The model under review builds one solid part; all positions refer to its coordinate system, in mm. Face numbers are marked on the shaded views. Coordinates: 2 decimals unless noted, no trailing zeros. Loops run counter-clockwise (first coordinate to the right, second up) from the corner with the lowest first, then second, coordinate; pieces in that order, holes last. Notation, with made-up numbers: (76.5, 54) - (91.5, 54) arc R19 cw to (91.5, 78) - close; hole circle Ø6 at (77.25, -13). An arc over 180 degrees is marked (long way). Use a Markdown table: item, result. Add a question column.
1) To check wall thickness, follow L1, parallel to Y at x = -21.25, z = -14.8; L2, parallel to Y at x = -264.45, z = -14.8; L3, parallel to X at y = 181.5, z = -10. State the ranges of each line that lie inside material, in increasing order. Write a range as [from, to].
2) Clearance check with flat-ended pins moving along their axes: pin 1 (2 mm diameter, centred on y = 182, z = -22.8, fed in from +X); pin 2 (1.1 mm diameter, centred on x = -21.5, y = 177, fed in from -Z); pin 3 (6 mm diameter, centred on x = -83.5, z = -5.5, fed in from +Y); pin 4 (12 mm diameter, centred on x = -177, y = 99.5, fed in from +Z). State where each tip first meets the part, or that it passes through.
3) Add section B-B, the plane y = 73. Give the boundary of the cut face in (x, z).
4) Add section A-A, the plane z = -35. Give the boundary of the cut face in (x, y), and give its area (3 significant figures).
5) The part is to be moulded in two halves that separate along X. For the marked faces 1, 2, 3 and 4, say which applies: pulls with the +X half, pulls with the -X half, needs draft (parallel to the pull), parting line crosses it, or undercut.
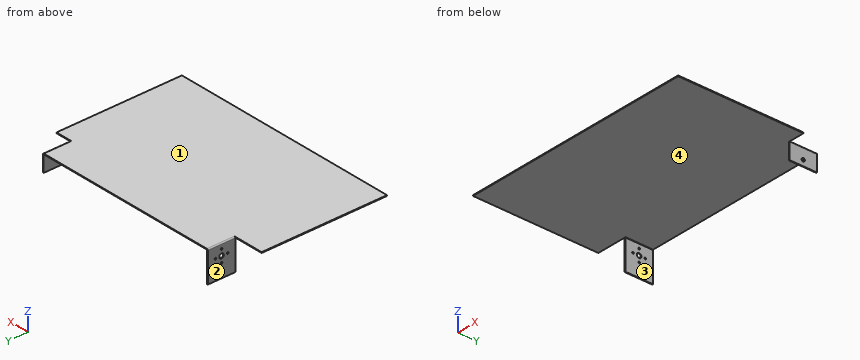
```python
from build123d import *

# Parameters (mm, degrees)
SKETCH1_W                    = 304
SKETCH1_H                    = 200
BASE_FLANGE1_DEPTH           = 1
SKETCH2_W                    = 39
SKETCH2_H                    = 36
CUT_EXTRUDE1_DEPTH           = 10
EDGE_FLANGE1_STRIP_W         = 5
EDGE_FLANGE1_STRIP_H         = 1
EDGE_FLANGE1_STRIP_CUT_DEPTH = 36
EDGE_FLANGE1_DEPTH           = 36
SKETCH9_R                    = 1.1
SKETCH9_R_2                  = 3
CUT_EXTRUDE2_DEPTH           = 10
CUT_EXTRUDE4_REACH           = 368.129
SKETCH18_W                   = 20.8
SKETCH18_H                   = 36
EDGE_FLANGE2_STRIP_W         = 5
EDGE_FLANGE2_STRIP_H         = 1
EDGE_FLANGE2_STRIP_CUT_DEPTH = 36
EDGE_FLANGE2_DEPTH           = 36
M4_CLEARANCE_HOLE2_D         = 4.3


# Sheet-metal steps are written as plain solids
with BuildPart() as part:
    # Sketch1 → Base-Flange1 (new body)
    with BuildSketch(Plane.XY):
        with Locations((-152, 100)):
            Rectangle(SKETCH1_W, SKETCH1_H)
    extrude(amount=-BASE_FLANGE1_DEPTH)

    # Sketch2 → Cut-Extrude1 (cut)
    with BuildSketch(Plane.XY):
        with Locations((-284.5, 182)):
            Rectangle(SKETCH2_W, SKETCH2_H)
    extrude(amount=-CUT_EXTRUDE1_DEPTH, mode=Mode.SUBTRACT)

    # Edge-Flange1 strip (across the edge) → Edge-Flange1 strip cut (cut)
    with BuildSketch(Plane(origin=(-265, 164, -1), x_dir=(1, 0, 0), z_dir=(0, 1, 0))):
        with Locations((-1, -0.5)):
            Rectangle(EDGE_FLANGE1_STRIP_W, EDGE_FLANGE1_STRIP_H)
    extrude(amount=EDGE_FLANGE1_STRIP_CUT_DEPTH, mode=Mode.SUBTRACT)

    # Edge-Flange1 section (across the edge) → Edge-Flange1 (add)
    with BuildSketch(Plane(origin=(-265, 164, -1), x_dir=(1, 0, 0), z_dir=(0, 1, 0))):
        with BuildLine():
            Line((0, 0.5), (0, 39.429))
            Line((0, 39.429), (1, 39.429))
            Line((1, 39.429), (1, 0.5))
            ThreePointArc((1, 0.5), (1.146446609, 0.146446609), (1.5, 0))
            Line((1.5, 0), (1.5, -1))
            ThreePointArc((1.5, -1), (0.439339828, -0.560660172), (0, 0.5))
        make_face()
    extrude(amount=EDGE_FLANGE1_DEPTH)

    # Sketch9 → Cut-Extrude2 (cut)
    with BuildSketch(Plane(origin=(-264, 0, 0), x_dir=(0, 0, -1), z_dir=(1, 0, 0))):
        with Locations((22.8, 182)):
            Circle(SKETCH9_R)
        with Locations((14.8, 190)):
            Circle(SKETCH9_R)
        with Locations((14.8, 174)):
            Circle(SKETCH9_R)
        with Locations((6.8, 182)):
            Circle(SKETCH9_R)
        with Locations((14.8, 182)):
            Circle(SKETCH9_R_2)
    extrude(amount=-CUT_EXTRUDE2_DEPTH, mode=Mode.SUBTRACT)

    # Sketch18 → Cut-Extrude4 (cut, up to next)
    with BuildSketch(Plane.XY, mode=Mode.PRIVATE) as cut_extrude4_sk1:
        with Locations((-10.4, 182)):
            Rectangle(SKETCH18_W, SKETCH18_H)
    cut_extrude4_tool1 = extrude(cut_extrude4_sk1.sketch, amount=-CUT_EXTRUDE4_REACH, mode=Mode.PRIVATE) & part.part
    add(cut_extrude4_tool1.solids().sort_by_distance((-10.4, 182, 0))[0], mode=Mode.SUBTRACT)

    # Edge-Flange2 strip (across the edge) → Edge-Flange2 strip cut (cut)
    with BuildSketch(Plane(origin=(-20.8, 200, -1), x_dir=(-1, 0, 0), z_dir=(0, -1, 0))):
        with Locations((-1, -0.5)):
            Rectangle(EDGE_FLANGE2_STRIP_W, EDGE_FLANGE2_STRIP_H)
    extrude(amount=EDGE_FLANGE2_STRIP_CUT_DEPTH, mode=Mode.SUBTRACT)

    # Edge-Flange2 section (across the edge) → Edge-Flange2 (add)
    with BuildSketch(Plane(origin=(-20.8, 200, -1), x_dir=(-1, 0, 0), z_dir=(0, -1, 0))):
        with BuildLine():
            Line((0, 0.5), (0, 21.2292))
            Line((0, 21.2292), (1, 21.2292))
            Line((1, 21.2292), (1, 0.5))
            ThreePointArc((1, 0.5), (1.146446609, 0.146446609), (1.5, 0))
            Line((1.5, 0), (1.5, -1))
            ThreePointArc((1.5, -1), (0.439339828, -0.560660172), (0, 0.5))
        make_face()
    extrude(amount=EDGE_FLANGE2_DEPTH)

    # M4 Clearance Hole2 (through all)
    with Locations(Plane.ZY.offset(21.8)):
        with Locations((-14.8, 182)):
            Hole(M4_CLEARANCE_HOLE2_D / 2)


solid = part.part
```
From the geometry:
| question | item | result |
|---|---|---|
| 1 | L1 | y = [164, 179.85], [184.15, 200] |
| 1 | L2 | y = [164, 172.9], [175.1, 179], [185, 188.9], [191.1, 200] |
| 1 | L3 | x = [-265, -264], [-21.8, -20.8] |
| 2 | pin 1 | stops at x = -20.8 |
| 2 | pin 2 | stops at z = -22.23 |
| 2 | pin 3 | passes through |
| 2 | pin 4 | stops at z = 0 |
| 3 | outline | (-304, -1) - (0, -1) - (0, 0) - (-304, 0) - close |
| 4 | outline | (-265, 164) - (-264, 164) - (-264, 200) - (-265, 200) - close |
| 4 | area | 36.0 mm^2 |
| 5 | face 1 | needs draft |
| 5 | face 2 | pulls with the -X half |
| 5 | face 3 | undercut |
| 5 | face 4 | undercut |
